Could you check a few things on this model? Use its own coordinates, in mm. A direction names the side the tool comes from. Give positions to 0.01 mm unless a question says otherwise; leave off trailing zeros. Write each loop counter-clockwise with the first axis right and the second up, starting at its lowest first coordinate (ties: lowest second). Pieces come first, ordered by that corner, then holes. Notation, with made-up numbers: (45.25, 65) - (54.25, 65) arc R14 cw to (54.25, 86) - close; hole circle Ø6 at (53.25, 50). An arc over 180 degrees is marked (long way). Answer as a JSON object with one key per item and string values. Group by question number.
```python
from build123d import *

# Parameters (mm, degrees)
SKETCH1_R           = 13.25
SKETCH1_R_2         = 1.3
SKETCH1_R_3         = 3.9
BOSS_EXTRUDE1_DEPTH = 3
BOSS_EXTRUDE2_DEPTH = 3


with BuildPart() as part:
    # Sketch1 → Boss-Extrude1 (new body)
    # profile 1 of 2: a face of its own
    with BuildSketch(Plane.XY):
        with Locations((0, 3.25)):
            Circle(SKETCH1_R)
        with Locations((8.5, 3.25)):
            Circle(SKETCH1_R_2, mode=Mode.SUBTRACT)
        with Locations((-8.5, 3.25)):
            Circle(SKETCH1_R_2, mode=Mode.SUBTRACT)
        with Locations((0, 3.25)):
            Circle(SKETCH1_R_3, mode=Mode.SUBTRACT)
    # profile 2 of 2: a face of its own
    with BuildSketch(Plane.XY):
        with BuildLine():
            Line((-13.25, 3.249999993), (-13.25, -16.5))
            Line((-13.25, -16.5), (13.25, -16.5))
            Line((13.25, -16.5), (13.25, 3.25))
            ThreePointArc((13.25, 3.25), (4e-09, -10), (-13.25, 3.249999993))
        make_face()
    extrude(amount=BOSS_EXTRUDE1_DEPTH)

    # Sketch2 → Boss-Extrude2 (add)
    with BuildSketch(Plane.XZ.offset(16.5)):
        with BuildLine():
            Line((0, 32.5), (-13.25, 32.5))
            Line((-13.25, 32.5), (-13.25, 3))
            Line((-13.25, 3), (0, 3))
            Line((0, 3), (0, 10.178644607))
            Line((0, 10.178644607), (-6.477335786, 10.178644607))
            ThreePointArc((-6.477335786, 10.178644607), (-9.037995958, 9.117984436), (-7.977335786, 11.678644607))
            Line((-7.977335786, 11.678644607), (-7.977335786, 23.821355393))
            ThreePointArc((-7.977335786, 23.821355393), (-9.037995958, 26.382015564), (-6.477335786, 25.321355393))
            Line((-6.477335786, 25.321355393), (0, 25.321355393))
            Line((0, 25.321355393), (0, 32.5))
        make_face()
        with BuildLine():
            Line((13.25, 32.5), (0, 32.5))
            Line((0, 32.5), (0, 25.321355393))
            Line((0, 25.321355393), (6.477335786, 25.321355393))
            ThreePointArc((6.477335786, 25.321355393), (7.977335786, 26.821355393), (9.477335786, 25.321355393))
            ThreePointArc((9.477335786, 25.321355393), (9.037995958, 24.260695221), (7.977335786, 23.821355393))
            Line((7.977335786, 23.821355393), (7.977335786, 11.678644607))
            ThreePointArc((7.977335786, 11.678644607), (9.037995958, 11.239304779), (9.477335786, 10.178644607))
            ThreePointArc((9.477335786, 10.178644607), (7.977335786, 8.678644607), (6.477335786, 10.178644607))
            Line((6.477335786, 10.178644607), (0, 10.178644607))
            Line((0, 10.178644607), (0, 3))
            Line((0, 3), (13.25, 3))
            Line((13.25, 3), (13.25, 32.5))
        make_face()
        with BuildLine():
            Line((6.477335786, 25.321355393), (0, 25.321355393))
            Line((0, 25.321355393), (0, 22.75))
            ThreePointArc((0, 22.75), (3.535533906, 21.285533906), (5, 17.75))
            ThreePointArc((5, 17.75), (3.535533906, 14.214466094), (0, 12.75))
            Line((0, 12.75), (0, 10.178644607))
            Line((0, 10.178644607), (6.477335786, 10.178644607))
            ThreePointArc((6.477335786, 10.178644607), (6.916675614, 11.239304779), (7.977335786, 11.678644607))
            Line((7.977335786, 11.678644607), (7.977335786, 23.821355393))
            ThreePointArc((7.977335786, 23.821355393), (6.916675614, 24.260695221), (6.477335786, 25.321355393))
        make_face()
        with BuildLine():
            Line((0, 22.75), (0, 25.321355393))
            Line((0, 25.321355393), (-6.477335786, 25.321355393))
            ThreePointArc((-6.477335786, 25.321355393), (-6.916675614, 24.260695221), (-7.977335786, 23.821355393))
            Line((-7.977335786, 23.821355393), (-7.977335786, 11.678644607))
            ThreePointArc((-7.977335786, 11.678644607), (-6.916675614, 11.239304779), (-6.477335786, 10.178644607))
            Line((-6.477335786, 10.178644607), (0, 10.178644607))
            Line((0, 10.178644607), (0, 12.75))
            ThreePointArc((0, 12.75), (-5, 17.75), (0, 22.75))
        make_face()
    extrude(amount=-BOSS_EXTRUDE2_DEPTH)


solid = part.part
```
(1) For faces 1 (the flat face through (13.25, -15, 10)), 2 (the flat face through (-6, -13.5, 18)), which set-ups out of +Z, -Z, +X, -X, +Y, -Y let a thin tool reach every point of the face, with its end or its side?
(2) I want a section at D-D, the plane z = 6. Please give me the cut outline in (x, y), and give its area (3 significant figures).
(3) Will these pins go through, and if not, where does the flat tip stop? P1, Ø3, axis at x = 5, y = 13, coming from the +Z side; P2, Ø3.5, axis at x = -7.98, z = 25.32, coming from the +Y side.
(4) I want a section at C-C, the plane y = -10. Please give me the cut outline in (x, z), and give its area (3 significant figures).
(5) I want a section at A-A, the plane z = 21. Please give me the cut outline in (x, y).
(6) If we mould it in two halves opening along Y, with no side actions, what happens to faces 3 (the cylindrical face through (-3.095, 0.877, 1.479)), 4 (the cylindrical face through (0.291, 16.497, 1.479)), 5 (the flat face through (0, -15, 32.5))? For each: +Y half, -Y half, draft (parallel to the pull), parting line (faces both ways), or undercut.
(7) I need wall thicknesses on L1, parallel to Y at x = 0, z = 1.25; L2, parallel to Y at x = 5.5, z = 11.5; L3, parallel to Z at x = 10.5, y = 6. Which ranges of each line are inside material? Lowest first, please.
(8) I want a section at B-B, the plane x = -3. Please give me the cut outline in (y, z), and give its area (3 significant figures).
Entries:
{
 "1": {"face 1": "+Z, -Z, +X, +Y, -Y", "face 2": "+Z, +X, -X, +Y"},
 "2": {"outline": "(-13.25, -16.5) - (13.25, -16.5) - (13.25, -13.5) - (-13.25, -13.5) - close", "area": "79.5 mm^2"},
 "3": {"P1": "z = 3", "P2": "y = -13.5"},
 "4": {"outline": "(-13.25, 0) - (13.25, 0) - (13.25, 3) - (-13.25, 3) - close", "area": "79.5 mm^2"},
 "5": {"outline": "(-13.25, -16.5) - (-3.8, -16.5) - (-3.8, -13.5) - (-13.25, -13.5) - close; (3.8, -16.5) - (13.25, -16.5) - (13.25, -13.5) - (3.8, -13.5) - close"},
 "6": {"face 3": "undercut", "face 4": "+Y half", "face 5": "draft"},
 "7": {"L1": "-16.5 to -0.65, 7.15 to 16.5", "L2": "-16.5 to -13.5", "L3": "0 to 3"},
 "8": {"outline": "(-16.5, 0) - (0.76, 0) - (0.76, 3) - (-13.5, 3) - (-13.5, 13.75) - (-16.5, 13.75) - close; (-16.5, 21.75) - (-13.5, 21.75) - (-13.5, 32.5) - (-16.5, 32.5) - close; (5.74, 0) - (16.16, 0) - (16.16, 3) - (5.74, 3) - close", "area": "148 mm^2"}
}
